Part model, mm, in its own coordinate system. Coordinates: 2 decimals unless noted, no trailing zeros. Order: outer loops, then holes, each group sorted by start corner. A loop starts at its lowest first (then second) coordinate and runs counter-clockwise, first axis right, second up.
```python
from build123d import *

# Parameters (mm, degrees)
EXTRUSION1_DEPTH         = 5
ENL_V_MAT_EXTRU_14_REACH = 176.146
ESQUISSE8_R              = 2


with BuildPart() as part:
    # Esquisse1 → Extrusion1 (new body)
    with BuildSketch(Plane(origin=(0, 0, 0), x_dir=(1, 0, 0), z_dir=(0, 1, 0))):
        Polygon((-64.179491924, 79.940798285), (98.820508076, 79.940798285), (103.820508076, 74.940798285), (103.820508076, 24.940798285), (101.320508076, 15.610671266), (19.820508076, -125.551469551), (12.990381057, -127.38159657), (-30.310889132, -102.38159657), (-37.141016151, -95.551469551), (-118.641016151, 45.610671266), (-116.810889132, 52.440798285), (-73.509618943, 77.440798285), align=None)
    extrude(amount=EXTRUSION1_DEPTH)

    # Esquisse8 → Enlèv. mat.-Extru.14 (cut, up to next)
    with BuildSketch(Plane(origin=(0, 5, 0), x_dir=(1, 0, 0), z_dir=(0, 1, 0)), mode=Mode.PRIVATE) as enl_v_mat_extru_14_sk1:
        with Locations(Location((-103.168584287, 32.81163316, 0), (0, 0, 270))):
            Circle(ESQUISSE8_R)
    enl_v_mat_extru_14_tool1 = extrude(enl_v_mat_extru_14_sk1.sketch, amount=-ENL_V_MAT_EXTRU_14_REACH, mode=Mode.PRIVATE) & part.part
    # Esquisse8 → Enlèv. mat.-Extru.14 (cut, up to next)
    with BuildSketch(Plane(origin=(0, 5, 0), x_dir=(1, 0, 0), z_dir=(0, 1, 0)), mode=Mode.PRIVATE) as enl_v_mat_extru_14_sk2:
        with Locations(Location((80, 72.940798285, 0), (0, 0, 270))):
            Circle(ESQUISSE8_R)
    enl_v_mat_extru_14_tool2 = extrude(enl_v_mat_extru_14_sk2.sketch, amount=-ENL_V_MAT_EXTRU_14_REACH, mode=Mode.PRIVATE) & part.part
    # Esquisse8 → Enlèv. mat.-Extru.14 (cut, up to next)
    with BuildSketch(Plane(origin=(0, 5, 0), x_dir=(1, 0, 0), z_dir=(0, 1, 0)), mode=Mode.PRIVATE) as enl_v_mat_extru_14_sk3:
        with Locations(Location((20, 72.940798285, 0), (0, 0, 270))):
            Circle(ESQUISSE8_R)
    enl_v_mat_extru_14_tool3 = extrude(enl_v_mat_extru_14_sk3.sketch, amount=-ENL_V_MAT_EXTRU_14_REACH, mode=Mode.PRIVATE) & part.part
    # Esquisse8 → Enlèv. mat.-Extru.14 (cut, up to next)
    with BuildSketch(Plane(origin=(0, 5, 0), x_dir=(1, 0, 0), z_dir=(0, 1, 0)), mode=Mode.PRIVATE) as enl_v_mat_extru_14_sk4:
        with Locations(Location((-73.168584287, -19.149891067, 0), (0, 0, 270))):
            Circle(ESQUISSE8_R)
    enl_v_mat_extru_14_tool4 = extrude(enl_v_mat_extru_14_sk4.sketch, amount=-ENL_V_MAT_EXTRU_14_REACH, mode=Mode.PRIVATE) & part.part
    # Esquisse8 → Enlèv. mat.-Extru.14 (cut, up to next)
    with BuildSketch(Plane(origin=(0, 5, 0), x_dir=(1, 0, 0), z_dir=(0, 1, 0)), mode=Mode.PRIVATE) as enl_v_mat_extru_14_sk5:
        with Locations(Location((-43.168584287, -71.111415294, 0), (0, 0, 270))):
            Circle(ESQUISSE8_R)
    enl_v_mat_extru_14_tool5 = extrude(enl_v_mat_extru_14_sk5.sketch, amount=-ENL_V_MAT_EXTRU_14_REACH, mode=Mode.PRIVATE) & part.part
    # Esquisse8 → Enlèv. mat.-Extru.14 (cut, up to next)
    with BuildSketch(Plane(origin=(0, 5, 0), x_dir=(1, 0, 0), z_dir=(0, 1, 0)), mode=Mode.PRIVATE) as enl_v_mat_extru_14_sk6:
        with Locations(Location((-40, 72.940798285, 0), (0, 0, 270))):
            Circle(ESQUISSE8_R)
    enl_v_mat_extru_14_tool6 = extrude(enl_v_mat_extru_14_sk6.sketch, amount=-ENL_V_MAT_EXTRU_14_REACH, mode=Mode.PRIVATE) & part.part
    # Esquisse8 → Enlèv. mat.-Extru.14 (cut, up to next)
    with BuildSketch(Plane(origin=(0, 5, 0), x_dir=(1, 0, 0), z_dir=(0, 1, 0)), mode=Mode.PRIVATE) as enl_v_mat_extru_14_sk7:
        with Locations(Location((23.168584287, -105.752431445, 0), (0, 0, 270))):
            Circle(ESQUISSE8_R)
    enl_v_mat_extru_14_tool7 = extrude(enl_v_mat_extru_14_sk7.sketch, amount=-ENL_V_MAT_EXTRU_14_REACH, mode=Mode.PRIVATE) & part.part
    # Esquisse8 → Enlèv. mat.-Extru.14 (cut, up to next)
    with BuildSketch(Plane(origin=(0, 5, 0), x_dir=(1, 0, 0), z_dir=(0, 1, 0)), mode=Mode.PRIVATE) as enl_v_mat_extru_14_sk8:
        with Locations(Location((53.168584287, -53.790907218, 0), (0, 0, 270))):
            Circle(ESQUISSE8_R)
    enl_v_mat_extru_14_tool8 = extrude(enl_v_mat_extru_14_sk8.sketch, amount=-ENL_V_MAT_EXTRU_14_REACH, mode=Mode.PRIVATE) & part.part
    # Esquisse8 → Enlèv. mat.-Extru.14 (cut, up to next)
    with BuildSketch(Plane(origin=(0, 5, 0), x_dir=(1, 0, 0), z_dir=(0, 1, 0)), mode=Mode.PRIVATE) as enl_v_mat_extru_14_sk9:
        with Locations(Location((83.168584287, -1.829382991, 0), (0, 0, 270))):
            Circle(ESQUISSE8_R)
    enl_v_mat_extru_14_tool9 = extrude(enl_v_mat_extru_14_sk9.sketch, amount=-ENL_V_MAT_EXTRU_14_REACH, mode=Mode.PRIVATE) & part.part
    add(enl_v_mat_extru_14_tool1.solids().sort_by_distance((-103.168584, 5, -32.811633))[0], mode=Mode.SUBTRACT)
    add(enl_v_mat_extru_14_tool2.solids().sort_by_distance((80, 5, -72.940798))[0], mode=Mode.SUBTRACT)
    add(enl_v_mat_extru_14_tool3.solids().sort_by_distance((20, 5, -72.940798))[0], mode=Mode.SUBTRACT)
    add(enl_v_mat_extru_14_tool4.solids().sort_by_distance((-73.168584, 5, 19.149891))[0], mode=Mode.SUBTRACT)
    add(enl_v_mat_extru_14_tool5.solids().sort_by_distance((-43.168584, 5, 71.111415))[0], mode=Mode.SUBTRACT)
    add(enl_v_mat_extru_14_tool6.solids().sort_by_distance((-40, 5, -72.940798))[0], mode=Mode.SUBTRACT)
    add(enl_v_mat_extru_14_tool7.solids().sort_by_distance((23.168584, 5, 105.752431))[0], mode=Mode.SUBTRACT)
    add(enl_v_mat_extru_14_tool8.solids().sort_by_distance((53.168584, 5, 53.790907))[0], mode=Mode.SUBTRACT)
    add(enl_v_mat_extru_14_tool9.solids().sort_by_distance((83.168584, 5, 1.829383))[0], mode=Mode.SUBTRACT)


solid = part.part
```
(1) Drop flat-ended pins along their axis: pin 1 (5 mm diameter, centred on x = 20, z = -72.94, fed in from -Y); pin 2 (1.5 mm diameter, centred on y = 3, z = 79, fed in from -X); pin 3 (2 mm diameter, centred on x = -70.5, y = 3.5, fed in from +Z). Give the stop position or say it passes through.
(2) Slice it at B-B, the plane x = -9.5. Give the cut face in (y, z).
(3) Probe line 1 (Z direction, x = 55, y = 0.5); line 2 (Z direction, x = -21, y = 2.4); line 3 (X direction, y = 1.05, z = -42.5). List the from-to ranges inside material, lowest first.
(4) Slice it at C-C, the plane z = -65.5. Give the cut face in (x, y), then the cut area to 3 significant figures.
(5) Slice it at A-A, the plane y = 1.2. State how many separate pieces and enclosed holes the cut face has, then the cut area to 3 significant figures.
Here are the results:
1. pin 1: stops at y = 0
1. pin 2: stops at x = -47.13
1. pin 3: stops at z = 39.5
2. outline: (0, -79.94) - (5, -79.94) - (5, 114.4) - (0, 114.4) - close
3. line 1: z = -79.94 to 52.99, 54.59 to 64.62
3. line 2: z = -79.94 to 107.76
3. line 3: x = -116.85 to 103.82
4. outline: (-94.19, 0) - (103.82, 0) - (103.82, 5) - (-94.19, 5) - close
4. area: 990 mm2
5. separate pieces: 1
5. enclosed holes: 9
5. area: 29,900 mm2
